Geometry: final body of the model. Coordinates: model frame, mm. A direction names the side the tool comes from. Give positions to 0.01 mm unless a question says otherwise; leave off trailing zeros. Order: outer loops, then holes, each group sorted by start corner. A loop starts at its lowest first (then second) coordinate and runs counter-clockwise, first axis right, second up. Notation, with made-up numbers: M 79.5,-23 L 129.5,-23 A33 cw 129.5,9 Z; hole C -6,80.25 d7. An arc over 180 degrees is marked long. One line per item, written item: value. Start each with the question number.
```python
from build123d import *

# Parameters (mm, degrees)
SKETCH_1_W          = 142
SKETCH_1_H          = 88
SKETCH_1_W_2        = 116
SKETCH_1_H_2        = 64
EXTRUDE_1_DEPTH     = 30
CUT_EXTRUDE_1_DEPTH = 117.982904734
SKETCH_4_W          = 64
SKETCH_4_H          = 16.727272727
CUT_EXTRUDE_2_DEPTH = 152.657508881
FILLET_3_R          = 4
CHAMFER_2_SIZE      = 14.5
CUT_EXTRUDE_4_REACH = 118.983
SKETCH_8_R          = 19.5
CUT_EXTRUDE_5_REACH = 118.983
SKETCH_9_R          = 24.5
F_4_X_M5_D          = 4.2
F_4_X_M5_2_D        = 5.3


with BuildPart() as part:
    # 草图1 → 凸台-拉伸1 (new body)
    with BuildSketch(Plane(origin=(0, 0, 0), x_dir=(1, 0, 0), z_dir=(0, 1, 0))):
        Rectangle(SKETCH_1_W, SKETCH_1_H)
        Rectangle(SKETCH_1_W_2, SKETCH_1_H_2, mode=Mode.SUBTRACT)
    extrude(amount=-EXTRUDE_1_DEPTH)

    # 草图2 → 切除-拉伸1 (cut, through all)
    with BuildSketch(Plane.XY.offset(44)):
        Polygon((71, -6), (38, -30), (71, -30), align=None)
        Polygon((-71, -30), (-71, -6), (-38, -30), align=None)
    extrude(amount=-CUT_EXTRUDE_1_DEPTH, mode=Mode.SUBTRACT)

    # 草图4 → 切除-拉伸2 (cut, through all)
    with BuildSketch(Plane.ZY.offset(71)):
        with Locations((0, -14.363636364)):
            Rectangle(SKETCH_4_W, SKETCH_4_H)
    extrude(amount=-CUT_EXTRUDE_2_DEPTH, mode=Mode.SUBTRACT)

    # 圆角3
    fillet_3_edges = [part.edges().sort_by_distance(p)[0] for p in [
        (58, -3, -32),
        (58, -3, 32),
        (-58, -3, 32),
        (-58, -3, -32),
    ]]
    fillet(fillet_3_edges, radius=FILLET_3_R)

    # 倒角2
    # the kernel refuses this chamfer: 14.5 mm, written as the material it takes off along each edge
    with BuildSketch(Plane(origin=(71, 37.289403326, 44), x_dir=(-0.9996219169112966, 0, 0.027495876610586445), z_dir=(0, -1, 0)), Plane(origin=(-71, 37.289403326, 44), x_dir=(-0.02749587661058598, 0, -0.9996219169112966), z_dir=(0, -1, 0)), Plane(origin=(-71, 37.289403326, -44), x_dir=(0.9996219169112966, 0, -0.027495876610586455), z_dir=(0, -1, 0))) as chamfer_2_piece_1:
        Polygon((CHAMFER_2_SIZE * 0.999621916911, CHAMFER_2_SIZE * 0.0274958766106), (-CHAMFER_2_SIZE * 0.0274958766106, CHAMFER_2_SIZE * 0.999621916911), (0, 0), align=None)
    extrude(amount=80.578806651, mode=Mode.SUBTRACT)
    with BuildSketch(Plane(origin=(71, 37.289403326, -44), x_dir=(-0.9996219169112966, 0, -0.027495876610586455), z_dir=(0, -1, 0))) as chamfer_2_piece_2:
        Polygon((CHAMFER_2_SIZE * 0.999621916911, -CHAMFER_2_SIZE * 0.0274958766106), (-CHAMFER_2_SIZE * 0.0274958766106, -CHAMFER_2_SIZE * 0.999621916911), (0, 0), align=None)
    extrude(amount=80.578806651, mode=Mode.SUBTRACT)

    # 草图8 → 切除-拉伸4 (cut, up to next)
    with BuildSketch(Plane.XY.offset(44), mode=Mode.PRIVATE) as cut_extrude_4_sk1:
        with Locations((0, -30)):
            Circle(SKETCH_8_R)
    cut_extrude_4_tool1 = extrude(cut_extrude_4_sk1.sketch, amount=-CUT_EXTRUDE_4_REACH, mode=Mode.PRIVATE) & part.part
    add(cut_extrude_4_tool1.solids().sort_by_distance((0, -30, 44))[0], mode=Mode.SUBTRACT)

    # 草图9 → 切除-拉伸5 (cut, up to next)
    with BuildSketch(Plane(origin=(0, 0, -44), x_dir=(-1, 0, 0), z_dir=(0, 0, -1)), mode=Mode.PRIVATE) as cut_extrude_5_sk1:
        with Locations((0, -30)):
            Circle(SKETCH_9_R)
    cut_extrude_5_tool1 = extrude(cut_extrude_5_sk1.sketch, amount=-CUT_EXTRUDE_5_REACH, mode=Mode.PRIVATE) & part.part
    add(cut_extrude_5_tool1.solids().sort_by_distance((0, -30, -44))[0], mode=Mode.SUBTRACT)

    # 4 x M5 (through all)
    with Locations(Plane(origin=(0, 0, 0), x_dir=(-1, 0, 0), z_dir=(0, 1, 0))):
        with Locations((30, -38), (-30, -38), (-30, 38), (30, 38)):
            Hole(F_4_X_M5_D / 2)

    # 4 x M5 2 (through all)
    with Locations(Plane(origin=(0, 0, 0), x_dir=(-1, 0, 0), z_dir=(0, 1, 0))):
        with Locations((65, -26), (-65, -26), (65, 26), (-65, 26)):
            Hole(F_4_X_M5_2_D / 2)


solid = part.part
```
Q1. Section query A-A on z = -9.5. Return loops of the section in (x, y).
Q2. Section query B-B on x = 30. Return loops of the section in (y, z), and give its area (3 significant figures).
Q3. Section query C-C on y = -25.5. Return loops of the section in (x, z), and give its area (3 significant figures).
Q4. Set-up query: faces 5 (the face through (33, -30, -38)), 6 (the face through (56.797, -3.042, 30.859)), 7 (the face through (-0.539, -5.506, -38.084)). Return all of +Z, -Z, +X, -X, +Y, -Y with unobstructed straight access to the full face (end or side cutting, diameter ignored); none if empty.
Q5. Ray query, line 1 along Z through (x, y) = (-30, -9.5); line 2 along X through (y, z) = (-2.5, 28); line 3 along X through (y, z) = (-4, -39). Return the intervals inside material, ascending. Write a range as [from, to].
Q6. Section query D-D on z = -26. Return loops of the section in (x, y).
Q7. Mould query, pull axis Z, two halves, no side actions, for faces 1 (the face through (-62.2, -6.3, 38.3)), 2 (the face through (67.528, -3.042, -25.204)), 3 (the face through (-71, -3, 0)), 4 (the face through (-1, -5, -32)). Classes: +Z half, -Z half, draft (parallel to the pull), parting line (faces both ways), or undercut.
Q8. Contact query for flat-ended pins moving along their axis: pin 1 (6 mm diameter, centred on x = 65, z = -26, fed in from -Y); pin 2 (5.5 mm diameter, centred on x = -30, z = 38, fed in from -Y); pin 3 (9 mm diameter, centred on x = -11.5, y = -15, fed in from -Z); pin 4 (12 mm diameter, centred on y = -13, z = 28, fed in from +X). Output: stop coordinate, or through.
Results below:
1. outline: M -71,-6 L -58,-6 L -58,0 L -71,0 Z; M 58,-6 L 71,-6 L 71,0 L 58,0 Z
2. outline: M -30,-44 L 0,-44 L 0,-40.1 L -30,-40.1 Z; M -30,-35.9 L 0,-35.9 L 0,-32 L -30,-32 Z; M -30,32 L 0,32 L 0,35.9 L -30,35.9 Z; M -30,40.1 L 0,40.1 L 0,44 L -30,44 Z
2. area: 468 mm2
3. outline: M -44.19,-44 L -24.08,-44 L -24.08,-32 L -44.19,-32 Z; M -44.19,32 L -18.97,32 L -18.97,44 L -44.19,44 Z; M 18.97,32 L 44.19,32 L 44.19,44 L 18.97,44 Z; M 24.08,-44 L 44.19,-44 L 44.19,-32 L 24.08,-32 Z; hole C -30,-38 d4.2; hole C -30,38 d4.2; hole C 30,-38 d4.2; hole C 30,38 d4.2
3. area: 1,030 mm2
4. face 5: +Z, -Z, +X, -X, -Y
4. face 6: +Y, -Y
4. face 7: -Z, -Y
5. line 1: [-44, -40.1], [-35.9, -32], [32, 35.9], [40.1, 44]
5. line 2: [-71, -66.74], [-63.26, -58], [58, 63.26], [66.74, 71]
5. line 3: [-61.5, -31.85], [-28.15, 28.15], [31.85, 61.5]
6. outline: M -71,-6 L -67.65,-6 L -67.65,0 L -71,0 Z; M -62.35,-6 L -58,-6 L -58,0 L -62.35,0 Z; M 58,-6 L 62.35,-6 L 62.35,0 L 58,0 Z; M 67.65,-6 L 71,-6 L 71,0 L 67.65,0 Z
7. face 1: +Z half
7. face 2: undercut
7. face 3: draft
7. face 4: undercut
8. pin 1: y = -6
8. pin 2: y = -30
8. pin 3: z = 32
8. pin 4: x = 67.52
